Source: CAD feature listing. Evaluate the final solid. Frame: model axes, mm. Round coordinates to 2 decimals unless told otherwise and drop trailing zeros. Loops run counter-clockwise (first coordinate to the right, second up) from the corner with the lowest first, then second, coordinate; pieces in that order, holes last. Notation, with made-up numbers: (-39.75, 71) - (-13.75, 71) arc R23 cw to (-13.75, 97) - close; hole circle Ø3 at (34, -27). An arc over 180 degrees is marked (long way). Write item = value, one per line. Start each with the question number.
from build123d import *

# Parameters (mm, degrees)
SKETCH1_R               = 31.75
BOSS_EXTRUDE3_DEPTH     = 850.9
SKETCH1_3_R             = 31.75
BOSS_EXTRUDE4_DEPTH     = 63.5
SKETCH5_R               = 31.75
BOSS_EXTRUDE5_DEPTH     = 63.5
CUT_EXTRUDE7_DEPTH      = 96.774
CUT_EXTRUDE7_DEPTH_BACK = 96.774


with BuildPart() as part:
    # Sketch1 → Boss-Extrude3 (new body)
    with BuildSketch(Plane(origin=(0, 0, 0), x_dir=(1, 0, 0), z_dir=(0, 1, 0))):
        Circle(SKETCH1_R)
    extrude(amount=BOSS_EXTRUDE3_DEPTH)

    # Sketch1_3 → Boss-Extrude4 (add)
    with BuildSketch(Plane(origin=(0, 0, 0), x_dir=(1, 0, 0), z_dir=(0, 1, 0))):
        Circle(SKETCH1_3_R)
    extrude(amount=-BOSS_EXTRUDE4_DEPTH)

    # Sketch5 → Boss-Extrude5 (add)
    with BuildSketch(Plane(origin=(0, 850.9, 0), x_dir=(1, 0, 0), z_dir=(0, 1, 0))):
        Circle(SKETCH5_R)
    extrude(amount=BOSS_EXTRUDE5_DEPTH)

    # Sketch2 → Cut-Extrude7 (cut, two sides)
    with BuildSketch(Plane.XY) as cut_extrude7_sk:
        Polygon((31.75, 850.9), (31.75, 914.4), (-31.75, 914.4), align=None)
        Polygon((31.75, -63.5), (-31.75, -63.5), (31.75, 0), align=None)
    extrude(amount=CUT_EXTRUDE7_DEPTH, mode=Mode.SUBTRACT)
    extrude(cut_extrude7_sk.sketch, amount=-CUT_EXTRUDE7_DEPTH_BACK, mode=Mode.SUBTRACT)


solid = part.part
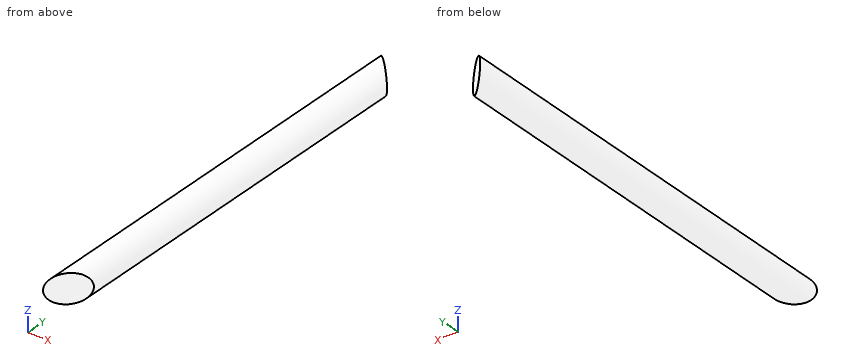
(1) Cut plane B-B (x = -5.5). Output: boundary loops of the cut face in (y, z), and give its area (3 significant figures).
(2) Cut plane C-C (y = 585.5). Output: boundary loops of the cut face in (x, z), and give its area (3 significant figures).
(3) Cut plane A-A (z = 0). Output: boundary loops of the cut face in (x, y), and give its area (3 significant figures).
(4) Material intervals for line 1 along Z through (x, y) = (1.5, 821); line 2 along Y through (x, z) = (11.5, -24.5), sorted ascending. Write a range as from..to.
(5) Pin query (flat end, axial travel): P1, Ø8, axis at x = -8.5, y = 726.5, coming from the -Z side; P2, Ø8, axis at y = 484, z = 12.5, coming from the -X side; P3, Ø6, axis at x = 23.5, y = 430, coming from the -Z side. Return the tip coordinate at first contact, or that it passes through.
Solution:
q1.outline = (-37.25, -31.27) - (888.15, -31.27) - (888.15, 31.27) - (-37.25, 31.27) - close
q1.area = 57,900 mm^2
q2.outline = circle Ø63.5 at (0, 0)
q2.area = 3,170 mm^2
q3.outline = (-31.75, -63.5) - (31.75, 0) - (31.75, 850.9) - (-31.75, 914.4) - close
q3.area = 58,100 mm^2
q4.line_1 = -31.71..31.71
q4.line_2 = -20.25..871.15
q5.P1 = -31.43
q5.P2 = -30.59
q5.P3 = -24.24
